Could you check a few things on this drawing? It's one solid part, dimensions in mm from its lowest x, y, z. Give positions to 0.01 mm unless a question says otherwise; leave off trailing zeros. Write each loop counter-clockwise with the first axis right and the second up, starting at its lowest first coordinate (ties: lowest second). Pieces come first, ordered by that corner, then holes. Notation, with made-up numbers: (39.25, 88.25) - (84.25, 88.25) arc R19 ccw to (84.25, 97.25) - close; hole circle Ø5 at (-18.5, 75). An arc over 180 degrees is marked (long way). One line per item, written item: value. Start each with the question number.
1) I'm going to push flat-ended pins straight in: P1, Ø3, axis at x = 23.5, y = 34.5, coming from the -Z side; P2, Ø12, axis at y = 41, z = 33.5, coming from the -X side; P3, Ø10, axis at y = 14.5, z = 13, coming from the +X side. Where does each tip first touch, or does it pass through?
2) Imagine slicing it at B-B on y = 42.5. Write out the boundary of the cut face in (x, z).
3) Imagine slicing it at A-A on y = 49.5. Write out the boundary of the cut face in (x, z).
4) We'd pull the mould along X, two halves only. Please class the marked faces 1, 2, 3 and 4: +X half, -X half, draft (parallel to the pull), parting line (faces both ways), or undercut.
5) Please list where these lines run through material, in increasing order: L1, parallel to X at y = 17, z = 40; L2, parallel to Y at x = 37, z = 45; L3, parallel to X at y = 43.5, z = 50. Write a range as [from, to].
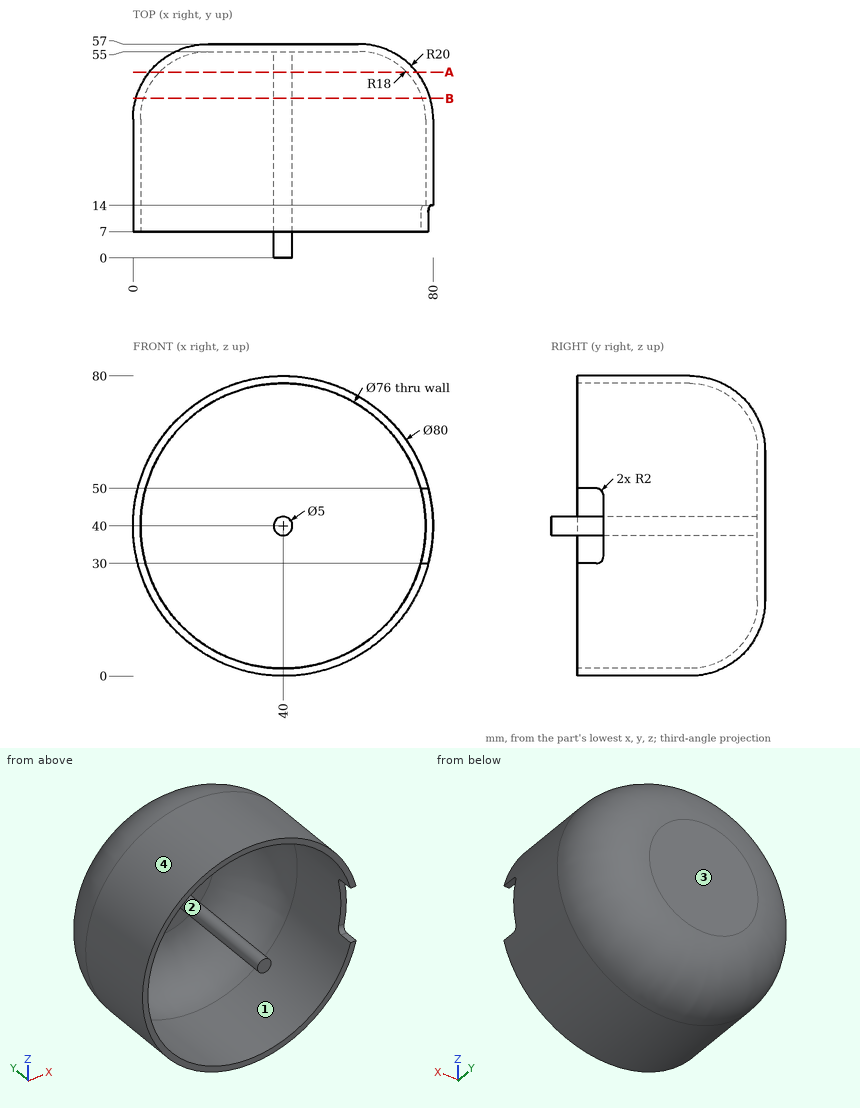
Numbers:
1. P1: z = 2.92
1. P2: x = 0.04
1. P3: x = 73.41
2. outline: circle Ø78.46 at (40, 40); circle Ø5 at (40, 40); hole circle Ø74.28 at (40, 40)
3. outline: circle Ø71.22 at (40, 40); circle Ø5 at (40, 40); hole circle Ø65.9 at (40, 40)
4. face 1: undercut
4. face 2: undercut
4. face 3: draft
4. face 4: parting line
5. L1: [0, 2], [37.5, 42.5], [78, 80]
5. L2: [55, 57]
5. L3: [2.39, 4.6], [75.4, 77.61]
